Work out the finished part from the listing and answer in its coordinate system (mm). A direction names the side the tool comes from. Coordinates: 2 decimals unless noted, no trailing zeros. Order: outer loops, then holes, each group sorted by start corner. A loop starts at its lowest first (then second) coordinate and runs counter-clockwise, first axis right, second up. Notation, with made-up numbers: (49, 24) - (104, 24) arc R23 cw to (104, 48) - close; hole circle Ø6 at (37.25, 24.25). An arc over 180 degrees is marked (long way). Answer as a JSON object with one key per item and string values. Group by question number.
1) Find the intervals of material crossed by line 1 along X through (y, z) = (2.5, 30); line 2 along Y through (x, z) = (-8, 34); line 3 along Y through (x, z) = (3.25, 31.5), in increasing order.
2) Section C-C (z = 6) is taken. Give the vertices of the cut face in (x, y).
3) Section A-A (x = 0) is taken. Give the vertices of the cut face in (y, z), plus the area to 3 significant figures.
4) The mould has two halves that part along X. Classify faces 4 (the face through (-3.47, 6.877, 33.001)), 5 (the face through (-9, 0, 20)): released by +X, released by -X, zero draft, split by the parting line, or undercut.
5) Section D-D (z = 30) is taken. Count the separate pieces of the cut face and the enclosed holes in it, plus the area to 3 significant figures.
6) A tool of negligible diameter and unlimited length cuts with its end or side. For faces 1 (the face through (-6.93, 2.87, 33)), 2 (the face through (-8.777, 7.822, 1.232)), 3 (the face through (0, 9, 20)), from which of +Z, -Z, +X, -X, +Y, -Y can it reach the whole face along a straight path? Write none if from no direction.
7) Each of these flat-tipped pins is pushed along its axis until it touches: P1, Ø5, axis at x = -0.5, z = 4, coming from the -Y side; P2, Ø2.5, axis at x = 0, y = 11, coming from the +Z side; P3, Ø1.8, axis at x = 11, y = 0, coming from the +Z side; P4, Ø12, axis at x = 3, z = 17.5, coming from the +Y side. Where does it stop, or does it pass through?
from build123d import *

# Parameters (mm, degrees)
CROQUIS1_R              = 13
CROQUIS1_R_2            = 1
SALIENTE_EXTRUIR1_DEPTH = 2.5
CROQUIS2_R              = 5
CORTAR_EXTRUIR2_DEPTH   = 2.5
SALIENTE_EXTRUIR2_START = 35.430987392
CROQUIS3_R              = 9
CROQUIS3_R_2            = 5
SALIENTE_EXTRUIR2_DEPTH = 35.430987392
SALIENTE_EXTRUIR3_REACH = 44.152
CROQUIS4_R              = 2.5
CROQUIS5_R              = 1
CORTAR_EXTRUIR3_DEPTH   = 10


with BuildPart() as part:
    # Croquis1 → Saliente-Extruir1 (new body)
    with BuildSketch(Plane.XY):
        Circle(CROQUIS1_R)
        with Locations((0, 11)):
            Circle(CROQUIS1_R_2, mode=Mode.SUBTRACT)
        with Locations((7.778174593, 7.778174593)):
            Circle(CROQUIS1_R_2, mode=Mode.SUBTRACT)
        with Locations((11, 0)):
            Circle(CROQUIS1_R_2, mode=Mode.SUBTRACT)
        with Locations((7.778174593, -7.778174593)):
            Circle(CROQUIS1_R_2, mode=Mode.SUBTRACT)
        with Locations((0, -11)):
            Circle(CROQUIS1_R_2, mode=Mode.SUBTRACT)
        with Locations((-7.778174593, -7.778174593)):
            Circle(CROQUIS1_R_2, mode=Mode.SUBTRACT)
        with Locations((-11, 0)):
            Circle(CROQUIS1_R_2, mode=Mode.SUBTRACT)
        with Locations((-7.778174593, 7.778174593)):
            Circle(CROQUIS1_R_2, mode=Mode.SUBTRACT)
    extrude(amount=SALIENTE_EXTRUIR1_DEPTH)

    # Croquis2 → Cortar-Extruir2 (cut)
    with BuildSketch(Plane.XY.offset(2.5)):
        Circle(CROQUIS2_R)
    extrude(amount=-CORTAR_EXTRUIR2_DEPTH, mode=Mode.SUBTRACT)

    # Croquis3 → Saliente-Extruir2 (add)
    with BuildSketch(Plane.XY.offset(2.5).offset(SALIENTE_EXTRUIR2_START)):
        with Locations(Location((0, 0, 0), (0, 0, 180))):
            Circle(CROQUIS3_R)
        Circle(CROQUIS3_R_2, mode=Mode.SUBTRACT)
    extrude(amount=-SALIENTE_EXTRUIR2_DEPTH)

    # Croquis4 → Saliente-Extruir3 (add, up to next)
    with BuildSketch(Plane.XY.offset(37.930987392), mode=Mode.PRIVATE) as saliente_extruir3_sk1:
        with Locations((3.444150891, 8.314915793)):
            Circle(CROQUIS4_R)
    saliente_extruir3_tool1 = extrude(saliente_extruir3_sk1.sketch, amount=-SALIENTE_EXTRUIR3_REACH, mode=Mode.PRIVATE) - part.part
    # Croquis4 → Saliente-Extruir3 (add, up to next)
    with BuildSketch(Plane.XY.offset(37.930987392), mode=Mode.PRIVATE) as saliente_extruir3_sk2:
        with Locations((8.314915793, 3.444150891)):
            Circle(CROQUIS4_R)
    saliente_extruir3_tool2 = extrude(saliente_extruir3_sk2.sketch, amount=-SALIENTE_EXTRUIR3_REACH, mode=Mode.PRIVATE) - part.part
    # Croquis4 → Saliente-Extruir3 (add, up to next)
    with BuildSketch(Plane.XY.offset(37.930987392), mode=Mode.PRIVATE) as saliente_extruir3_sk3:
        with Locations((8.314915793, -3.444150891)):
            Circle(CROQUIS4_R)
    saliente_extruir3_tool3 = extrude(saliente_extruir3_sk3.sketch, amount=-SALIENTE_EXTRUIR3_REACH, mode=Mode.PRIVATE) - part.part
    # Croquis4 → Saliente-Extruir3 (add, up to next)
    with BuildSketch(Plane.XY.offset(37.930987392), mode=Mode.PRIVATE) as saliente_extruir3_sk4:
        with Locations((3.444150891, -8.314915793)):
            Circle(CROQUIS4_R)
    saliente_extruir3_tool4 = extrude(saliente_extruir3_sk4.sketch, amount=-SALIENTE_EXTRUIR3_REACH, mode=Mode.PRIVATE) - part.part
    # Croquis4 → Saliente-Extruir3 (add, up to next)
    with BuildSketch(Plane.XY.offset(37.930987392), mode=Mode.PRIVATE) as saliente_extruir3_sk5:
        with Locations((-3.444150891, -8.314915793)):
            Circle(CROQUIS4_R)
    saliente_extruir3_tool5 = extrude(saliente_extruir3_sk5.sketch, amount=-SALIENTE_EXTRUIR3_REACH, mode=Mode.PRIVATE) - part.part
    # Croquis4 → Saliente-Extruir3 (add, up to next)
    with BuildSketch(Plane.XY.offset(37.930987392), mode=Mode.PRIVATE) as saliente_extruir3_sk6:
        with Locations((-8.314915793, -3.444150891)):
            Circle(CROQUIS4_R)
    saliente_extruir3_tool6 = extrude(saliente_extruir3_sk6.sketch, amount=-SALIENTE_EXTRUIR3_REACH, mode=Mode.PRIVATE) - part.part
    # Croquis4 → Saliente-Extruir3 (add, up to next)
    with BuildSketch(Plane.XY.offset(37.930987392), mode=Mode.PRIVATE) as saliente_extruir3_sk7:
        with Locations((-8.314915793, 3.444150891)):
            Circle(CROQUIS4_R)
    saliente_extruir3_tool7 = extrude(saliente_extruir3_sk7.sketch, amount=-SALIENTE_EXTRUIR3_REACH, mode=Mode.PRIVATE) - part.part
    # Croquis4 → Saliente-Extruir3 (add, up to next)
    with BuildSketch(Plane.XY.offset(37.930987392), mode=Mode.PRIVATE) as saliente_extruir3_sk8:
        with Locations((-3.444150891, 8.314915793)):
            Circle(CROQUIS4_R)
    saliente_extruir3_tool8 = extrude(saliente_extruir3_sk8.sketch, amount=-SALIENTE_EXTRUIR3_REACH, mode=Mode.PRIVATE) - part.part
    add(saliente_extruir3_tool1.solids().sort_by_distance((3.444151, 8.314916, 37.930987))[0])
    add(saliente_extruir3_tool2.solids().sort_by_distance((8.314916, 3.444151, 37.930987))[0])
    add(saliente_extruir3_tool3.solids().sort_by_distance((8.314916, -3.444151, 37.930987))[0])
    add(saliente_extruir3_tool4.solids().sort_by_distance((3.444151, -8.314916, 37.930987))[0])
    add(saliente_extruir3_tool5.solids().sort_by_distance((-3.444151, -8.314916, 37.930987))[0])
    add(saliente_extruir3_tool6.solids().sort_by_distance((-8.314916, -3.444151, 37.930987))[0])
    add(saliente_extruir3_tool7.solids().sort_by_distance((-8.314916, 3.444151, 37.930987))[0])
    add(saliente_extruir3_tool8.solids().sort_by_distance((-3.444151, 8.314916, 37.930987))[0])

    # Croquis5 → Cortar-Extruir3 (cut)
    with BuildSketch(Plane.XY.offset(37.930987392)):
        with Locations((-3.252809175, 7.852976026)):
            Circle(CROQUIS5_R)
        with Locations((3.252809175, 7.852976026)):
            Circle(CROQUIS5_R)
        with Locations((7.852976026, 3.252809175)):
            Circle(CROQUIS5_R)
        with Locations((7.852976026, -3.252809175)):
            Circle(CROQUIS5_R)
        with Locations((3.252809175, -7.852976026)):
            Circle(CROQUIS5_R)
        with Locations((-3.252809175, -7.852976026)):
            Circle(CROQUIS5_R)
        with Locations((-7.852976026, -3.252809175)):
            Circle(CROQUIS5_R)
        with Locations((-7.852976026, 3.252809175)):
            Circle(CROQUIS5_R)
    extrude(amount=-CORTAR_EXTRUIR3_DEPTH, mode=Mode.SUBTRACT)


solid = part.part
Report:
{
 "1": {"line 1": "x = -10.63 to -8.51, -7.19 to -4.33, 4.33 to 7.19, 8.51 to 10.63", "line 2": "y = -5.92 to -4.24, -2.26 to 2.26, 4.24 to 5.92", "line 3": "y = -10.81 to -8.85, -6.85 to -3.8, 3.8 to 6.85, 8.85 to 10.81"},
 "2": {"outline": "(-8.94, -1.02) arc R2.5 ccw (long way) to (-7.05, -5.6) arc R9 ccw to (-5.6, -7.05) arc R2.5 ccw (long way) to (-1.02, -8.94) arc R9 ccw to (1.02, -8.94) arc R2.5 ccw (long way) to (5.6, -7.05) arc R9 ccw to (7.05, -5.6) arc R2.5 ccw (long way) to (8.94, -1.02) arc R9 ccw to (8.94, 1.02) arc R2.5 ccw (long way) to (7.05, 5.6) arc R9 ccw to (5.6, 7.05) arc R2.5 ccw (long way) to (1.02, 8.94) arc R9 ccw to (-1.02, 8.94) arc R2.5 ccw (long way) to (-5.6, 7.05) arc R9 ccw to (-7.05, 5.6) arc R2.5 ccw (long way) to (-8.94, 1.02) arc R9 ccw to start; hole circle Ø10 at (0, 0)"},
 "3": {"outline": "(-13, 0) - (-12, 0) - (-12, 2.5) - (-13, 2.5) - close; (-10, 0) - (-5, 0) - (-5, 37.93) - (-9, 37.93) - (-9, 2.5) - (-10, 2.5) - close; (5, 0) - (10, 0) - (10, 2.5) - (9, 2.5) - (9, 37.93) - (5, 37.93) - close; (12, 0) - (13, 0) - (13, 2.5) - (12, 2.5) - close", "area": "313 mm²"},
 "4": {"face 4": "undercut", "face 5": "released by -X"},
 "5": {"separate pieces": "1", "enclosed holes": "9", "area": "234 mm²"},
 "6": {"face 1": "+Z", "face 2": "+Z, -Z", "face 3": "+Z, +Y"},
 "7": {"P1": "stops at y = -13", "P2": "stops at z = 2.5", "P3": "passes through", "P4": "stops at y = 10.81"}
}
